Could you check a few things on this model? Use its own coordinates, in mm. A direction names the side the tool comes from. Round coordinates to 2 decimals unless told otherwise and drop trailing zeros. Write each loop counter-clockwise with the first axis right and the second up, starting at its lowest first coordinate (ties: lowest second). Pieces come first, ordered by that corner, then holes. Notation, with made-up numbers: (22.25, -14.5) -> (67.25, -14.5) arc R21 cw to (67.25, -10.5) -> close; hole circle Ø1 at (56.25, -18). An arc over 180 degrees is marked (long way). Answer as CSV lines item,"result". Start each with the question number.
Q1. Imagine slicing it at C-C on x = 97.5. Give the number of separate pieces and of enclosed holes in the cut face, and give its area (3 significant figures).
Q2. Imagine slicing it at A-A on y = 42.5. Please give me the cut outline in (x, z), and give its area (3 significant figures).
Q3. Imagine slicing it at B-B on x = 134. Please give me the cut outline in (y, z).
Q4. For faces 4 (the flat face through (103.6, 28.035, 1.521)), 5 (the flat face through (73.209, 30, 1)), which set-ups out of +Z, -Z, +X, -X, +Y, -Y let a thin tool reach every point of the face, with its end or its side?
Q5. Imagine slicing it at D-D on y = 106. Please give me the cut outline in (x, z).
Q6. Will these pins go through, and if not, where does the flat tip stop? pin 1 Ø0.5 at (x, z) = (111, 1.5) entering from +Y; pin 2 Ø1.4 at (x, z) = (88, 1.5) entering from +Y; pin 3 Ø1.4 at (x, z) = (140.5, 1.5) entering from +Y.
Q7. If I drill on line 1 (X direction, y = 42, z = 2.3); line 2 (X direction, y = 31, z = 2.85); line 3 (X direction, y = 24.5, z = 0.55), over which ranges is the centre line in solid material (lowest first)? Write a range as [from, to].
Q8. If we mould it in two halves opening along X, with no side actions, what happens to faces 1 (the flat face through (114, 0, 1)), 2 (the flat face through (95, 10.404, 2)), 3 (the flat face through (153.209, 65, 1))? For each: pulls with the +X half, pulls with the -X half, needs draft (parallel to the pull), parting line crosses it, or undercut.
from build123d import *

# Parameters (mm, degrees)
BOSS_EXTRUDE1_DEPTH = 3
CUT_EXTRUDE1_DEPTH  = 3


with BuildPart() as part:
    # Sketch1 → Boss-Extrude1 (new body)
    with BuildSketch(Plane.XY):
        Polygon((73.208888624, 61.429551443), (153.208888624, 128.557521937), (153.208888624, 0), (73.208888624, 0), align=None)
    extrude(amount=BOSS_EXTRUDE1_DEPTH)

    # Sketch2 → Cut-Extrude1 (cut)
    with BuildSketch(Plane.XY.offset(3)):
        with BuildLine():
            Line((114.541115695, 24.848188193), (124.897018473, 50.403743749))
            Line((124.897018473, 50.403743749), (141.32931014, 50.403743749))
            Line((141.32931014, 50.403743749), (141.32931014, 49.292632638))
            Line((141.32931014, 49.292632638), (140.053268473, 49.292632638))
            add(Edge.make_bspline(
                [(140.053268473, 49.292632638), (139.777913916, 49.287279798), (139.250682366, 49.277030519), (138.50450005, 49.164580552), (137.836795314, 48.980086144), (137.446503851, 48.781055794), (137.258129584, 48.684993749)],
                knots=[0, 0, 0, 0, 1.141675553, 2.186008389, 3.124476521, 4, 4, 4, 4], degree=3))
            add(Edge.make_bspline(
                [(137.258129584, 48.684993749), (137.138546651, 48.611673708), (136.896313732, 48.463153122), (136.596086342, 48.143316904), (136.306505192, 47.77978632), (136.167514751, 47.49054629), (136.09493514, 47.339507638)],
                knots=[0, 0, 0, 0, 0.92689117, 1.877555159, 2.891677582, 4, 4, 4, 4], degree=3))
            add(Edge.make_bspline(
                [(136.09493514, 47.339507638), (136.066604666, 47.270746405), (136.002068988, 47.114111084), (135.953061058, 46.830507124), (135.885354455, 46.485384284), (135.848925671, 46.066688386), (135.81416284, 45.583570509), (135.785726516, 45.030780096), (135.783396388, 44.408347319), (135.777079325, 43.968548261), (135.773754584, 43.737077082)],
                knots=[0, 0, 0, 0, 0.489997979, 1.116195674, 1.892481991, 2.815045661, 3.888305079, 5.094018216, 6.470549178, 8, 8, 8, 8], degree=3))
            Line((135.773754584, 43.737077082), (135.773754584, 17.070410415))
            add(Edge.make_bspline(
                [(135.773754584, 17.070410415), (135.777068496, 16.836044569), (135.783409978, 16.387563484), (135.785856575, 15.750682405), (135.813746186, 15.183392289), (135.849629159, 14.68588278), (135.884629459, 14.25556917), (135.954037997, 13.89602331), (136.002450601, 13.601431222), (136.111395778, 13.306263295), (136.290115509, 12.990352676), (136.581751189, 12.649113903), (136.961506114, 12.339403102), (137.415488976, 12.049727482), (137.954119231, 11.806372313), (138.580490143, 11.635507838), (139.288825096, 11.531956263), (139.789572455, 11.520754017), (140.053268473, 11.51485486)],
                knots=[0, 0, 0, 0, 1.348866943, 2.581183741, 3.664677528, 4.616142033, 5.452864999, 6.145451543, 6.723473748, 7.165912693, 7.948706057, 8.799395909, 9.733211935, 10.758727886, 11.891513365, 13.119773514, 14.483258592, 16, 16, 16, 16], degree=3))
            Line((140.053268473, 11.51485486), (141.32931014, 11.51485486))
            Line((141.32931014, 11.51485486), (141.32931014, 10.403743749))
            Line((141.32931014, 10.403743749), (120.773754584, 10.403743749))
            Line((120.773754584, 10.403743749), (120.773754584, 11.51485486))
            Line((120.773754584, 11.51485486), (122.049796251, 11.51485486))
            add(Edge.make_bspline(
                [(122.049796251, 11.51485486), (122.328100051, 11.519788417), (122.855467853, 11.52913719), (123.603877097, 11.645167884), (124.268464025, 11.825399233), (124.659288026, 12.020932183), (124.84493514, 12.113813193)],
                knots=[0, 0, 0, 0, 1.154913481, 2.188486767, 3.139504729, 4, 4, 4, 4], degree=3))
            add(Edge.make_bspline(
                [(124.84493514, 12.113813193), (124.963688543, 12.187882908), (125.205993367, 12.339014992), (125.522548533, 12.651091277), (125.789467027, 13.038073651), (125.933569987, 13.327111023), (126.008129584, 13.476660415)],
                knots=[0, 0, 0, 0, 0.919236091, 1.875612259, 2.900831081, 4, 4, 4, 4], degree=3))
            add(Edge.make_bspline(
                [(126.008129584, 13.476660415), (126.036482482, 13.545417481), (126.101069242, 13.70204331), (126.149089491, 13.982919397), (126.218719843, 14.324814277), (126.253857147, 14.740845033), (126.289303378, 15.226779271), (126.316933013, 15.779620532), (126.319830601, 16.402028189), (126.326027204, 16.838937549), (126.32931014, 17.070410415)],
                knots=[0, 0, 0, 0, 0.491154816, 1.118830903, 1.878082211, 2.802823963, 3.878617243, 5.106317376, 6.466938293, 8, 8, 8, 8], degree=3))
            Line((126.32931014, 17.070410415), (126.32931014, 46.51485486))
            Line((126.32931014, 46.51485486), (111.633129584, 10.403743749))
            Line((111.633129584, 10.403743749), (110.956046251, 10.403743749))
            Line((110.956046251, 10.403743749), (96.034171251, 46.167632638))
            Line((96.034171251, 46.167632638), (96.034171251, 18.181521526))
            add(Edge.make_bspline(
                [(96.034171251, 18.181521526), (96.033190657, 17.958710944), (96.031318524, 17.533324619), (96.043902342, 16.928659169), (96.047406401, 16.39312255), (96.069662028, 15.924639846), (96.080811254, 15.524733601), (96.111073311, 15.192481376), (96.131378595, 14.927855243), (96.160396628, 14.77570005), (96.17306014, 14.709299304)],
                knots=[0, 0, 0, 0, 1.537276861, 2.934943876, 4.172912213, 5.231790959, 6.170977958, 6.931994631, 7.533920913, 8, 8, 8, 8], degree=3))
            add(Edge.make_bspline(
                [(96.17306014, 14.709299304), (96.24207751, 14.479788853), (96.378508228, 14.02610197), (96.742519421, 13.413991548), (97.187520669, 12.855403415), (97.757425274, 12.365276459), (98.475961448, 11.965325093), (99.371323366, 11.71141388), (100.422324645, 11.533357851), (101.183703417, 11.521290215), (101.589726807, 11.51485486)],
                knots=[0, 0, 0, 0, 0.837202277, 1.654947254, 2.477083681, 3.333000774, 4.272846669, 5.334753209, 6.578693578, 8, 8, 8, 8], degree=3))
            Line((101.589726807, 11.51485486), (101.589726807, 10.403743749))
            Line((101.589726807, 10.403743749), (87.700837918, 10.403743749))
            Line((87.700837918, 10.403743749), (87.700837918, 11.51485486))
            Line((87.700837918, 11.51485486), (88.108824029, 11.51485486))
            add(Edge.make_bspline(
                [(88.108824029, 11.51485486), (88.326119555, 11.515958146), (88.753567478, 11.518128449), (89.380690167, 11.601723744), (89.986576932, 11.729328159), (90.561772547, 11.920334861), (91.096566285, 12.153779677), (91.557403695, 12.449291329), (91.967729934, 12.754532224), (92.297594099, 13.128470853), (92.579118316, 13.5527757), (92.820072335, 14.047801623), (93.041761578, 14.61157873), (93.142726903, 15.023158324), (93.195629584, 15.238813193)],
                knots=[0, 0, 0, 0, 1.126221598, 2.215421052, 3.275368575, 4.333933395, 5.355119513, 6.292312747, 7.169137372, 7.998144275, 8.864108371, 9.803942606, 10.849334424, 12, 12, 12, 12], degree=3))
            add(Edge.make_bspline(
                [(93.195629584, 15.238813193), (93.202214921, 15.276348515), (93.219826457, 15.376731332), (93.220721213, 15.565972366), (93.23219697, 15.826075335), (93.239616075, 16.156072479), (93.248148475, 16.55823406), (93.259127372, 17.03274832), (93.255551074, 17.582569372), (93.256100465, 17.973190342), (93.256393473, 18.181521526)],
                knots=[0, 0, 0, 0, 0.310187739, 0.829552458, 1.537439513, 2.433908972, 3.518989584, 4.816276497, 6.302014132, 8, 8, 8, 8], degree=3))
            Line((93.256393473, 18.181521526), (93.256393473, 43.737077082))
            add(Edge.make_bspline(
                [(93.256393473, 43.737077082), (93.253065361, 43.971441664), (93.246696704, 44.419920331), (93.244433013, 45.05681769), (93.215819555, 45.626940178), (93.181647654, 46.124609011), (93.144463395, 46.554666597), (93.077514309, 46.908858762), (93.026352876, 47.199976304), (92.918911223, 47.492567379), (92.740012849, 47.808500991), (92.448251073, 48.149453568), (92.067439137, 48.462006467), (91.607344322, 48.747016559), (91.066151715, 48.990534713), (90.439896314, 49.17604788), (89.726495128, 49.273958557), (89.223100805, 49.286215027), (88.959518473, 49.292632638)],
                knots=[0, 0, 0, 0, 1.347272511, 2.578132646, 3.660345685, 4.627277135, 5.446463535, 6.138231406, 6.69929032, 7.141206279, 7.92307434, 8.772758631, 9.705470838, 10.743855472, 11.875301939, 13.106723778, 14.485051461, 16, 16, 16, 16], degree=3))
            Line((88.959518473, 49.292632638), (87.700837918, 49.292632638))
            Line((87.700837918, 49.292632638), (87.700837918, 50.403743749))
            Line((87.700837918, 50.403743749), (103.942157362, 50.403743749))
            Line((103.942157362, 50.403743749), (114.541115695, 24.848188193))
        make_face()
    extrude(amount=-CUT_EXTRUDE1_DEPTH, mode=Mode.SUBTRACT)


solid = part.part
Checks:
1,separate pieces,"3"
1,enclosed holes,"0"
1,area,"216 mm^2"
2,outline,"(73.21, 0) -> (93.26, 0) -> (93.26, 3) -> (73.21, 3) -> close; (96.03, 0) -> (97.56, 0) -> (97.56, 3) -> (96.03, 3) -> close; (107.22, 0) -> (121.69, 0) -> (121.69, 3) -> (107.22, 3) -> close; (124.7, 0) -> (126.33, 0) -> (126.33, 3) -> (124.7, 3) -> close; (135.77, 0) -> (153.21, 0) -> (153.21, 3) -> (135.77, 3) -> close"
2,area,"165 mm^2"
3,outline,"(0, 0) -> (10.4, 0) -> (10.4, 3) -> (0, 3) -> close; (50.4, 0) -> (112.44, 0) -> (112.44, 3) -> (50.4, 3) -> close"
4,face 4,"+Z, -Z"
4,face 5,"+Z, -Z, -X, +Y, -Y"
5,outline,"(126.33, 0) -> (153.21, 0) -> (153.21, 3) -> (126.33, 3) -> close"
6,pin 1,"y = 93.35"
6,pin 2,"y = 74.43"
6,pin 3,"y = 118.48"
7,line 1,"[73.21, 93.26], [96.03, 97.77], [107.43, 121.49], [124.49, 126.33], [135.77, 153.21]"
7,line 2,"[73.21, 93.26], [96.03, 102.36], [111.99, 117.03], [120.02, 126.33], [135.77, 153.21]"
7,line 3,"[73.21, 93.26], [96.03, 105.07], [117.37, 126.33], [135.77, 153.21]"
8,face 1,"needs draft"
8,face 2,"undercut"
8,face 3,"pulls with the +X half"
